Source: three-view drawing plus pictorial views. Frame: mm from the lowest corner of the part. Give positions to 0.01 mm unless a question says otherwise; leave off trailing zeros. Loops run counter-clockwise (first coordinate to the right, second up) from the corner with the lowest first, then second, coordinate; pieces in that order, holes last. Notation, with made-up numbers: (69.5, 84.5) - (82.5, 84.5) arc R34 ccw to (82.5, 120.5) - close; hole circle Ø8 at (8, 28.5). An arc over 180 degrees is marked (long way). Put each result on its own line as item: value.
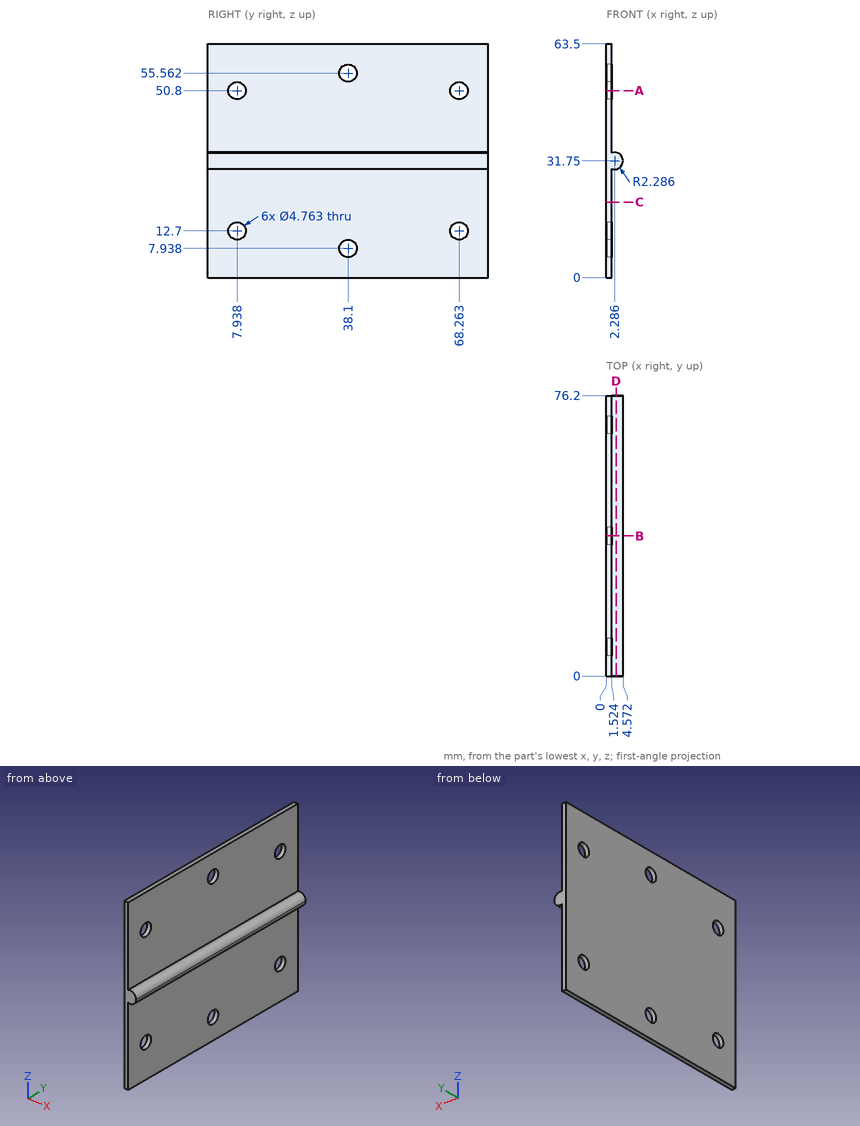
1) Material intervals for line 1 along Z through (x, y) = (0.45, 38.1); line 2 along X through (y, z) = (62.5, 28) (1 decimal); line 3 along Z through (x, y) = (2.2, 67.5) (1 decimal), sorted ascending. Write a range as [from, to].
Check result:
line 1: [0, 5.56], [10.32, 53.18], [57.94, 63.5]
line 2: [0, 1.5]
line 3: [29.5, 34]
2) Section query A-A, the plane z = 50.8. Output: boundary loops of the cut face in (x, y) (1 decimal).
Check result:
outline: (0, 0) - (1.5, 0) - (1.5, 5.6) - (0, 5.6) - close; (0, 10.3) - (1.5, 10.3) - (1.5, 65.9) - (0, 65.9) - close; (0, 70.6) - (1.5, 70.6) - (1.5, 76.2) - (0, 76.2) - close
3) Section query C-C, the plane z = 20.5. Output: boundary loops of the cut face in (x, y) (1 decimal).
Check result:
outline: (0, 0) - (1.5, 0) - (1.5, 76.2) - (0, 76.2) - close
4) Pin query (flat end, axial travel): P1, Ø7.5, axis at y = 7.94, z = 50.8, coming from the +X side. Return the tip coordinate at first contact, or that it passes through.
Check result:
P1: x = 1.52
5) Section query D-D, the plane x = 2.65. Output: boundary loops of the cut face in (y, z), plus the area to 3 significant figures.
Check result:
outline: (0, 29.49) - (76.2, 29.49) - (76.2, 34.01) - (0, 34.01) - close
area: 344 mm²
6) Section query B-B, the plane y = 38.1. State how many separate pieces and enclosed holes the cut face has.
Check result:
separate pieces: 3
enclosed holes: 0
